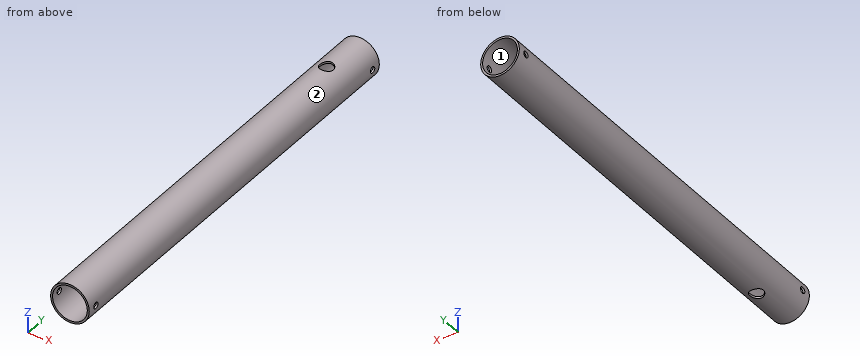
```python
from build123d import *

# Parameters (mm, degrees)
SKETCH1_R            = 10
SKETCH1_R_2          = 9
BOSS_EXTRUDE1_DEPTH  = 217
M3_CLEARANCE_HOLE1_D = 3.2
CUT_EXTRUDE1_REACH   = 22
SKETCH4_R            = 3.5
CUT_EXTRUDE2_REACH   = 22
SKETCH5_R            = 3.5


with BuildPart() as part:
    # Sketch1 → Boss-Extrude1 (new body)
    with BuildSketch(Plane(origin=(0, 0, 0), x_dir=(1, 0, 0), z_dir=(0, 1, 0))):
        Circle(SKETCH1_R)
        Circle(SKETCH1_R_2, mode=Mode.SUBTRACT)
    extrude(amount=BOSS_EXTRUDE1_DEPTH)

    # M3 Clearance Hole1 (through all)
    with Locations(Plane.ZY.offset(10)):
        with Locations((0, 5)):
            m3_clearance_hole1 = Hole(M3_CLEARANCE_HOLE1_D / 2)

    # Mirror1: M3 Clearance Hole1 across plane
    add(m3_clearance_hole1.mirror(Plane.ZX.offset(108.5)), mode=Mode.SUBTRACT)

    # Sketch4 → Cut-Extrude1 (cut, up to next)
    with BuildSketch(Plane(origin=(0, 0, -10), x_dir=(-1, 0, 0), z_dir=(0, 0, -1)), mode=Mode.PRIVATE) as cut_extrude1_sk1:
        with Locations((0, 25)):
            Circle(SKETCH4_R)
    cut_extrude1_tool1 = extrude(cut_extrude1_sk1.sketch, amount=-CUT_EXTRUDE1_REACH, mode=Mode.PRIVATE) & part.part
    add(cut_extrude1_tool1.solids().sort_by_distance((0, 25, -10))[0], mode=Mode.SUBTRACT)

    # Sketch5 → Cut-Extrude2 (cut, up to next)
    with BuildSketch(Plane.XY.offset(10), mode=Mode.PRIVATE) as cut_extrude2_sk1:
        with Locations((0, 192)):
            Circle(SKETCH5_R)
    cut_extrude2_tool1 = extrude(cut_extrude2_sk1.sketch, amount=-CUT_EXTRUDE2_REACH, mode=Mode.PRIVATE) & part.part
    add(cut_extrude2_tool1.solids().sort_by_distance((0, 192, 10))[0], mode=Mode.SUBTRACT)


solid = part.part
```
For this review, take the finished solid that the model builds, in its own axes (mm). Face numbers are marked on the shaded views. Coordinates: 2 decimals unless noted, no trailing zeros. Loops run counter-clockwise (first coordinate to the right, second up) from the corner with the lowest first, then second, coordinate; pieces in that order, holes last. Notation, with made-up numbers: (68.5, 56) -> (127.5, 56) arc R28 ccw to (127.5, 90) -> close; hole circle Ø11 at (67.25, 71.5). An arc over 180 degrees is marked (long way). Return JSON: item names as keys, results as strings. Group by question number.
(1) Consider section B-B, the plane z = -4.25. Give the boundary of the cut face in (x, y).
(2) To check wall thickness, follow L1, parallel to Y at x = -9.7, z = 0; L2, parallel to X at y = 130, z = 0; L3, parallel to Z at x = 1.25, y = 183. State the ranges of each line that lie inside material, in increasing order.
(3) Mouldability with a two-part tool opening along X and no side actions: class the marked faces 1 and 2 as pulls with the +X half, pulls with the -X half, needs draft (parallel to the pull), parting line crosses it, or undercut.
(4) Consider section A-A, the plane x = 0. Give the boundary of the cut face in (y, z).
(5) For pin 1 Ø1.9 at (y, z) = (5, 0) entering from +X; pin 2 Ø4 at (x, y) = (0, 25) entering from -Z; pin 3 Ø1.5 at (x, y) = (-7.5, 23) entering from +Z; pin 4 Ø8 at (y, z) = (22.5, 6.5) entering from +X, all flat-tipped, find the tip position at first contact; note any pin that passes through.
(6) Consider section C-C, the plane y = 141. Give the boundary of the cut face in (x, z), plus the area to 3 significant figures.
(7) Consider section D-D, the plane y = 25. Give the boundary of the cut face in (x, z).
Results below:
{
 "1": {"outline": "(-9.05, 0) -> (-7.93, 0) -> (-7.93, 217) -> (-9.05, 217) -> close; (7.93, 0) -> (9.05, 0) -> (9.05, 217) -> (7.93, 217) -> close"},
 "2": {"L1": "y = 0 to 3.4, 6.6 to 210.4, 213.6 to 217", "L2": "x = -10 to -9, 9 to 10", "L3": "z = -9.92 to -8.91, 8.91 to 9.92"},
 "3": {"face 1": "undercut", "face 2": "parting line crosses it"},
 "4": {"outline": "(0, -10) -> (21.5, -10) -> (21.5, -9) -> (0, -9) -> close; (0, 9) -> (188.5, 9) -> (188.5, 10) -> (0, 10) -> close; (28.5, -10) -> (217, -10) -> (217, -9) -> (28.5, -9) -> close; (195.5, 9) -> (217, 9) -> (217, 10) -> (195.5, 10) -> close"},
 "5": {"pin 1": "passes through", "pin 2": "stops at z = 8.77", "pin 3": "stops at z = 7.38", "pin 4": "stops at x = 9.68"},
 "6": {"outline": "circle Ø20 at (0, 0); hole circle Ø18 at (0, 0)", "area": "59.7 mm2"},
 "7": {"outline": "(-3.5, -9.37) -> (-3.5, -8.29) arc R9 cw (long way) to (3.5, -8.29) -> (3.5, -9.37) arc R10 ccw (long way) to start"}
}
